```python
from build123d import *

# Parameters (mm, degrees)
CROQUIS1_R              = 19.05
SALIENTE_EXTRUIR1_DEPTH = 185
CROQUIS2_W              = 0.838589864
CROQUIS2_H              = 1.125731298
CROQUIS2_W_2            = 0.770363726
CROQUIS2_W_3            = 1.091618228
CROQUIS2_H_2            = 0.62827213
CROQUIS2_H_3            = 0.668024516
SALIENTE_EXTRUIR2_DEPTH = 3


with BuildPart() as part:
    # Croquis1 → Saliente-Extruir1 (new body)
    with BuildSketch(Plane.XY):
        Circle(CROQUIS1_R)
    extrude(amount=SALIENTE_EXTRUIR1_DEPTH)

    # Croquis2 → Saliente-Extruir2 (add)
    with BuildSketch(Plane(origin=(0, 0, 0), x_dir=(-1, 0, 0), z_dir=(0, 0, -1))):
        with Locations((-19.05, 0)):
            Rectangle(CROQUIS2_W, CROQUIS2_H)
        with Locations((19.05, 0)):
            Rectangle(CROQUIS2_W_2, CROQUIS2_H)
        with Locations((0, 19.05)):
            Rectangle(CROQUIS2_W_3, CROQUIS2_H_2)
        with Locations((0, -19.05)):
            Rectangle(CROQUIS2_W_3, CROQUIS2_H_3)
    extrude(amount=-SALIENTE_EXTRUIR2_DEPTH)


solid = part.part
```
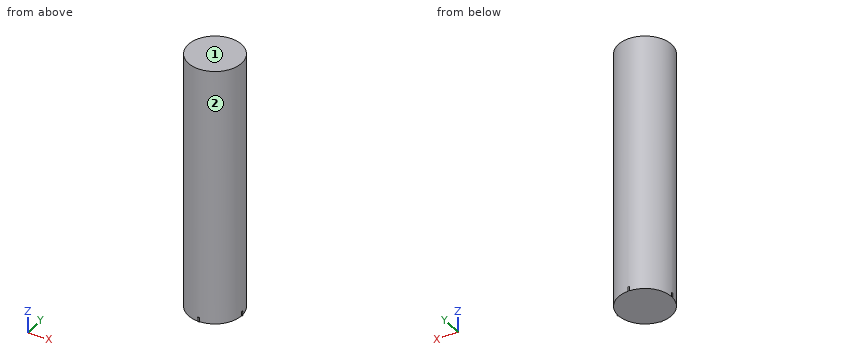
The listing builds one solid part. Answer for the finished solid, in the listing's coordinates (mm). Face numbers are marked on the shaded views. Coordinates: 2 decimals unless noted, no trailing zeros. Write each loop counter-clockwise with the first axis right and the second up, starting at its lowest first coordinate (ties: lowest second). Pieces come first, ordered by that corner, then holes. Notation, with made-up numbers: (67.5, 58) - (111.5, 58) arc R20 cw to (111.5, 64) - close; hole circle Ø10 at (86.5, 54). An arc over 180 degrees is marked (long way). Return JSON: item names as keys, results as strings. Group by question number.
1. A cutting plane is placed at B-B, the plane x = 9. Determine the outline of the cut face in (y, z).
2. Straight lines are drawn through the part: L1, parallel to X at y = 1, z = 19; L2, parallel to Y at x = 0, z = 85; L3, parallel to X at y = -4, z = 94.5. For each, find the intervals that lie inside material, in ascending order.
3. A cutting plane is placed at A-A, the plane z = 87.5. Determine the outline of the cut face in (x, y).
4. Given pin 1 (8 mm diameter, centred on x = 1.5, z = 60, fed in from +Y); pin 2 (5 mm diameter, centred on y = -2.5, z = 129, fed in from +X); pin 3 (6 mm diameter, centred on x = -11, z = 68, fed in from +Y), each flat-ended and moving along its own axis, determine where each tip first touches the part or whether it passes through.
5. A cutting plane is placed at C-C, the plane x = -2.5. Determine the outline of the cut face in (y, z).
6. Determine the mould class of the marked faces 1 and 2 for opening direction X: released by +X, released by -X, zero draft, split by the parting line, or undercut.
Ans:
{
 "1": {"outline": "(-16.79, 0) - (16.79, 0) - (16.79, 185) - (-16.79, 185) - close"},
 "2": {"L1": "-19.02 to 19.02", "L2": "-19.05 to 19.05", "L3": "-18.63 to 18.63"},
 "3": {"outline": "circle Ø38.1 at (0, 0)"},
 "4": {"pin 1": "y = 19.05", "pin 2": "x = 19.05", "pin 3": "y = 17.29"},
 "5": {"outline": "(-18.89, 0) - (18.89, 0) - (18.89, 185) - (-18.89, 185) - close"},
 "6": {"face 1": "zero draft", "face 2": "split by the parting line"}
}
